Answer from the drawing. Dimensions are ordinates in mm from the lowest x, y and z of the part. A direction names the side the tool comes from. Coordinates: 2 decimals unless noted, no trailing zeros. Write each loop counter-clockwise with the first axis right and the second up, starting at its lowest first coordinate (ties: lowest second). Pieces come first, ordered by that corner, then holes. Notation, with made-up numbers: M 33,4 L 78,4 A28 ccw 78,29 Z; hole C 34.25,59.25 d3. An arc over 180 degrees is marked long. Put each result on its own line as item: value. Start each with the question number.
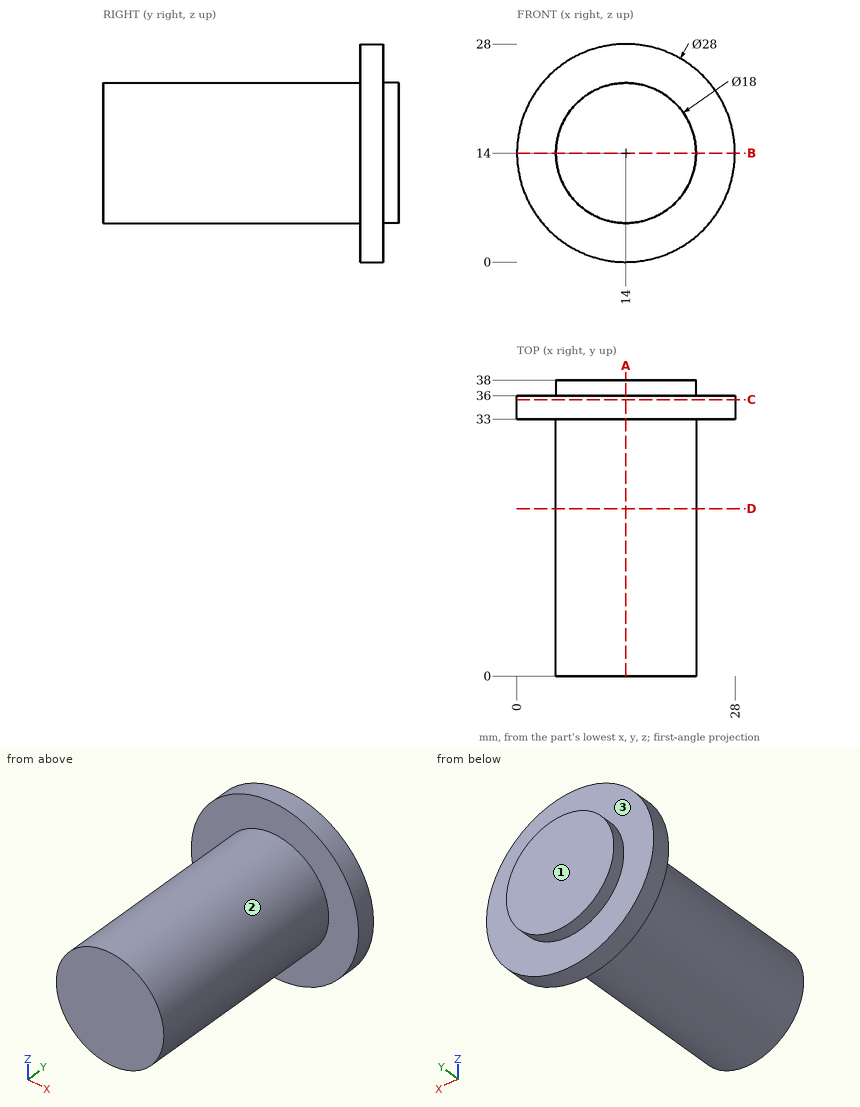
1) For the marked faces 1, 2 and 3, determine the directions among +Z, -Z, +X, -X, +Y, -Y from which every point of the face is accessible in a straight line to the end or side of a thin tool.
2) A cutting plane is placed at C-C on y = 35.5. Write down the section's boundary in (x, z), then the cut area to 3 significant figures.
3) A cutting plane is placed at A-A on x = 14. Write down the section's boundary in (y, z).
4) Given pin 1 Ø6 at (x, y) = (24, 9) entering from -Z; pin 2 Ø8 at (y, z) = (34, 8.5) entering from -X; pin 3 Ø12 at (x, y) = (21, 16.5) entering from -Z, each flat-ended and moving along its own axis, determine where each tip first touches the part or whether it passes through.
5) Straight lines are drawn through the part: probe 1 along Y at (x, z) = (2.5, 20.5); probe 2 along Z at (x, y) = (16.5, 11.5); probe 3 along X at (y, z) = (11.5, 12.5). For each, find the intervals that lie inside material, in ascending order.
6) A cutting plane is placed at B-B on z = 14. Write down the section's boundary in (x, y), then the cut area to 3 significant figures.
7) A cutting plane is placed at D-D on y = 21.5. Write down the section's boundary in (x, z), then the cut area to 3 significant figures.
Answers follow:
1. face 1: +Z, -Z, +X, -X, +Y
1. face 2: -Y
1. face 3: +Y
2. outline: C 14,14 d28
2. area: 616 mm²
3. outline: M 0,5 L 33,5 L 33,0 L 36,0 L 36,5 L 38,5 L 38,23 L 36,23 L 36,28 L 33,28 L 33,23 L 0,23 Z
4. pin 1: stops at z = 8.34
4. pin 2: stops at x = 0.08
4. pin 3: stops at z = 5.06
5. probe 1: y = 33 to 36
5. probe 2: z = 5.35 to 22.65
5. probe 3: x = 5.13 to 22.87
6. outline: M 0,33 L 5,33 L 5,0 L 23,0 L 23,33 L 28,33 L 28,36 L 23,36 L 23,38 L 5,38 L 5,36 L 0,36 Z
6. area: 714 mm²
7. outline: C 14,14 d18
7. area: 254 mm²
